```python
from build123d import *

# Parameters (mm, degrees)
SKETCH1_W           = 42.926
SKETCH1_H           = 42.926
SKETCH1_R           = 1.397
BOSS_EXTRUDE1_DEPTH = 2.54
SKETCH2_R           = 3.175
SKETCH2_R_2         = 1.397
BOSS_EXTRUDE2_DEPTH = 6.35
SKETCH3_R           = 3.175
SKETCH3_R_2         = 1.27
BOSS_EXTRUDE3_DEPTH = 6.35
SKETCH4_R           = 1.27
CUT_EXTRUDE1_DEPTH  = 9.89


with BuildPart() as part:
    # Sketch1 → Boss-Extrude1 (new body)
    with BuildSketch(Plane(origin=(0, 0, 0), x_dir=(1, 0, 0), z_dir=(0, 1, 0))):
        with Locations((-27.382131523, -2.193417639)):
            Rectangle(SKETCH1_W, SKETCH1_H)
        with Locations((-45.670131523, 16.094582361)):
            Circle(SKETCH1_R, mode=Mode.SUBTRACT)
        with Locations((-9.094131523, 16.094582361)):
            Circle(SKETCH1_R, mode=Mode.SUBTRACT)
        with Locations((-45.670131523, -20.481417639)):
            Circle(SKETCH1_R, mode=Mode.SUBTRACT)
        with Locations((-9.094131523, -20.481417639)):
            Circle(SKETCH1_R, mode=Mode.SUBTRACT)
    extrude(amount=BOSS_EXTRUDE1_DEPTH)

    # Sketch2 → Boss-Extrude2 (add)
    with BuildSketch(Plane(origin=(0, 2.54, 0), x_dir=(1, 0, 0), z_dir=(0, 1, 0))):
        with Locations((-45.670131523, 16.094582361)):
            Circle(SKETCH2_R)
        with Locations((-45.670131523, 16.094582361)):
            Circle(SKETCH2_R_2, mode=Mode.SUBTRACT)
        with Locations((-9.094131523, 16.094582361)):
            Circle(SKETCH2_R)
        with Locations((-9.094131523, 16.094582361)):
            Circle(SKETCH2_R_2, mode=Mode.SUBTRACT)
        with Locations((-9.094131523, -20.481417639)):
            Circle(SKETCH2_R)
        with Locations((-9.094131523, -20.481417639)):
            Circle(SKETCH2_R_2, mode=Mode.SUBTRACT)
        with Locations((-45.670131523, -20.481417639)):
            Circle(SKETCH2_R)
        with Locations((-45.670131523, -20.481417639)):
            Circle(SKETCH2_R_2, mode=Mode.SUBTRACT)
    extrude(amount=BOSS_EXTRUDE2_DEPTH)

    # Sketch3 → Boss-Extrude3 (add)
    with BuildSketch(Plane.XZ):
        with Locations((-32.462131523, 7.273417639)):
            Circle(SKETCH3_R)
        with Locations((-32.462131523, 7.273417639)):
            Circle(SKETCH3_R_2, mode=Mode.SUBTRACT)
        with Locations((-22.302131523, 7.273417639)):
            Circle(SKETCH3_R)
        with Locations((-22.302131523, 7.273417639)):
            Circle(SKETCH3_R_2, mode=Mode.SUBTRACT)
        with Locations((-22.302131523, -2.886582361)):
            Circle(SKETCH3_R)
        with Locations((-22.302131523, -2.886582361)):
            Circle(SKETCH3_R_2, mode=Mode.SUBTRACT)
        with Locations((-32.462131523, -2.886582361)):
            Circle(SKETCH3_R)
        with Locations((-32.462131523, -2.886582361)):
            Circle(SKETCH3_R_2, mode=Mode.SUBTRACT)
    extrude(amount=BOSS_EXTRUDE3_DEPTH)

    # Sketch4 → Cut-Extrude1 (cut, through all)
    with BuildSketch(Plane.XZ):
        with Locations((-32.462131523, -2.886582361)):
            Circle(SKETCH4_R)
        with Locations((-32.462131523, 7.273417639)):
            Circle(SKETCH4_R)
        with Locations((-22.302131523, -2.886582361)):
            Circle(SKETCH4_R)
        with Locations((-22.302131523, 7.273417639)):
            Circle(SKETCH4_R)
    extrude(amount=-CUT_EXTRUDE1_DEPTH, mode=Mode.SUBTRACT)


solid = part.part
```
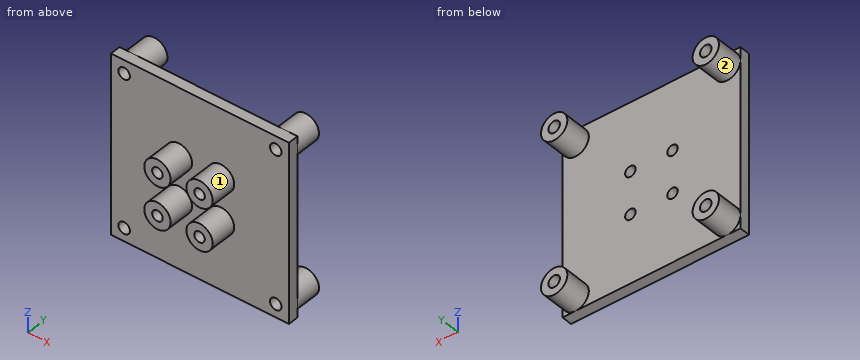
Source: CAD feature listing. Evaluate the final solid. Frame: model axes, mm. Face numbers are marked on the shaded views. A direction names the side the tool comes from. Round coordinates to 2 decimals unless told otherwise and drop trailing zeros. Loops run counter-clockwise (first coordinate to the right, second up) from the corner with the lowest first, then second, coordinate; pieces in that order, holes last.
(1) Section query D-D (y = -3.5). Output: boundary loops of the cut face in (x, z) (3 decimals), and give its area (3 significant figures).
From the geometry:
outline: circle Ø6.35 at (-32.462, -2.887); circle Ø6.35 at (-32.462, 7.273); circle Ø6.35 at (-22.302, -2.887); circle Ø6.35 at (-22.302, 7.273); hole circle Ø2.54 at (-32.462, -2.887); hole circle Ø2.54 at (-32.462, 7.273); hole circle Ø2.54 at (-22.302, -2.887); hole circle Ø2.54 at (-22.302, 7.273)
area: 106 mm2
(2) Material intervals for probe 1 along X at (y, z) = (0.75, 20.5); probe 2 along Z at (x, y) = (-32, -0.5); probe 3 along Y at (x, z) = (-27, -16.5), sorted ascending.
From the geometry:
probe 1: x = -48.85 to -47.07, -44.27 to -10.49, -7.7 to -5.92
probe 2: z = -6.03 to -4.07, -1.7 to 0.25, 4.13 to 6.09, 8.46 to 10.41
probe 3: y = 0 to 2.54
(3) Contact query for flat-ended pins moving along their axis: pin 1 Ø3.5 at (x, z) = (-32.46, -2.89) entering from +Y; pin 2 Ø4 at (x, y) = (-27, 6) entering from -Z; pin 3 Ø3 at (x, z) = (-9.09, 20.48) entering from -Y. Output: stop coordinate, or through.
From the geometry:
pin 1: stops at y = 2.54
pin 2: passes through
pin 3: stops at y = 0
(4) Section query B-B (x = -30). Output: boundary loops of the cut face in (y, z), and give its area (3 significant figures).
From the geometry:
outline: (-6.35, -4.89) - (0, -4.89) - (0, -19.27) - (2.54, -19.27) - (2.54, 23.66) - (0, 23.66) - (0, 9.28) - (-6.35, 9.28) - (-6.35, 5.27) - (0, 5.27) - (0, -0.88) - (-6.35, -0.88) - close
area: 160 mm2
(5) Section query C-C (z = 5). Output: boundary loops of the cut face in (x, y).
From the geometry:
outline: (-48.85, 0) - (-34.68, 0) - (-34.68, -6.35) - (-30.25, -6.35) - (-30.25, 0) - (-24.52, 0) - (-24.52, -6.35) - (-20.09, -6.35) - (-20.09, 0) - (-5.92, 0) - (-5.92, 2.54) - (-48.85, 2.54) - close
(6) Section query A-A (y = 5.25). Output: boundary loops of the cut face in (x, z) (3 decimals), and give its area (3 significant figures).
From the geometry:
outline: circle Ø6.35 at (-45.67, -16.095); circle Ø6.35 at (-45.67, 20.481); circle Ø6.35 at (-9.094, -16.095); circle Ø6.35 at (-9.094, 20.481); hole circle Ø2.794 at (-45.67, -16.095); hole circle Ø2.794 at (-45.67, 20.481); hole circle Ø2.794 at (-9.094, -16.095); hole circle Ø2.794 at (-9.094, 20.481)
area: 102 mm2
(7) Access query for the marked faces 1 and 2. Directions: +Z, -Z, +X, -X, +Y, -Y. A direction counts if a zero-diameter tool reaches every point of the face in a straight line with its end or side. Return the directions, or none.
From the geometry:
face 1: -Y
face 2: +Y
